```python
from build123d import *

# Parameters (mm, degrees)
SKETCH1_R           = 4.7625
BOSS_EXTRUDE1_DEPTH = 3.175
FILLET1_R           = 9.525


with BuildPart() as part:
    # Sketch1 → Boss-Extrude1 (new body)
    with BuildSketch(Plane.XY):
        Polygon((-195.314090033, 382.203190117), (-13.335, 248.156621006), (-13.335, 382.231468598), (-131.291653964, 469.118839915), align=None)
        with Locations((-35.56, 302.837639338)):
            Circle(SKETCH1_R, mode=Mode.SUBTRACT)
        with Locations((-35.56, 347.287639338)):
            Circle(SKETCH1_R, mode=Mode.SUBTRACT)
        with BuildLine():
            ThreePointArc((-154.070332508, 400.720749088), (-154.902423133, 400.218314877), (-155.846074695, 400.451417162))
            Line((-155.846074695, 400.451417162), (-161.470028505, 404.594045378))
            ThreePointArc((-161.470028505, 404.594045378), (-161.972462717, 405.426136003), (-161.739360431, 406.369787565))
            Line((-161.739360431, 406.369787565), (-129.351539832, 450.338880992))
            ThreePointArc((-129.351539832, 450.338880992), (-128.519449207, 450.841315204), (-127.575797645, 450.608212918))
            Line((-127.575797645, 450.608212918), (-121.951843834, 446.465584702))
            ThreePointArc((-121.951843834, 446.465584702), (-121.449409623, 445.633494077), (-121.682511908, 444.689842516))
            Line((-121.682511908, 444.689842516), (-154.070332508, 400.720749088))
        make_face(mode=Mode.SUBTRACT)
        Polygon((-150.783558745, 373.062079232), (-109.357276582, 429.301617336), (-54.61, 388.974541337), (-54.61, 302.220228189), (-96.036282162, 332.735003232), align=None, mode=Mode.SUBTRACT)
    extrude(amount=BOSS_EXTRUDE1_DEPTH)

    # Fillet1
    fillet1_edges = [part.edges().sort_by_distance(p)[0] for p in [
        (-54.61, 388.974541337, 1.5875),
        (-109.357276582, 429.301617336, 1.5875),
        (-150.783558745, 373.062079232, 1.5875),
        (-54.61, 302.220228189, 1.5875),
        (-131.291653964, 469.118839915, 1.5875),
        (-13.335, 382.231468598, 1.5875),
        (-13.335, 248.156621006, 1.5875),
        (-195.314090033, 382.203190117, 1.5875),
    ]]
    fillet(fillet1_edges, radius=FILLET1_R)


solid = part.part
```
Build history of the part. All positions in model axes, mm. A direction names the side the tool comes from. Round coordinates to 2 decimals unless told otherwise and drop trailing zeros. Write each loop counter-clockwise with the first axis right and the second up, starting at its lowest first coordinate (ties: lowest second). Pieces come first, ordered by that corner, then holes. Notation, with made-up numbers: (89, -18.75) - (128, -18.75) arc R23 cw to (128, -7.75) - close; hole circle Ø1 at (-24.5, -22.75). An arc over 180 degrees is marked (long way). Write each question's results on one line, items separated by ' | '. Start each with the question number.
Item 1: Drop a flat-ended pin along its axis: P1, Ø1.5, axis at x = -77.5, z = 1.5, coming from the +Y side. Give the stop position or say it passes through.
Item 2: Saw through at C-C (z = 2.5). State how many separate pieces and enclosed holes the cut face has, and give its area (3 significant figures).
Item 3: Saw through at B-B (x = -35.56). Write the cut outline in (y, z) (1 decimal), and give its area (3 significant figures).
Item 4: Which spindle directions (+Z, -Z, +X, -X, +Y, -Y) get a long thin tool onto all of the face, cutting with end or side? Do faces 1 (the face through (-158.619, 402.494, 1.565)), 2 (the face through (-18.695, 258.437, 1.61)). Say none if no direction does.
Item 5: Saw through at A-A (y = 364.5). Write the cut outline in (x, z) (3 decimals), and give its area (3 significant figures).
Item 6: Wall check: L1, parallel to X at y = 413, z = 1.4; L2, parallel to Y at x = -35.56, z = 0.9; L3, parallel to Y at x = -35, z = 2. Give the ranges that are in metal, low to high. Write a range as [from, to].
Results are:
1) P1: stops at y = 430.05
2) separate pieces: 1 | enclosed holes: 4 | area: 12,900 mm²
3) outline: (264.5, 0) - (298.1, 0) - (298.1, 3.2) - (264.5, 3.2) - close; (307.6, 0) - (342.5, 0) - (342.5, 3.2) - (307.6, 3.2) - close; (352.1, 0) - (398.6, 0) - (398.6, 3.2) - (352.1, 3.2) - close | area: 365 mm²
4) face 1: +Z, -Z | face 2: +Z, -Z, -Y
5) outline: (-171.281, 0) - (-139.16, 0) - (-139.16, 3.175) - (-171.281, 3.175) - close; (-54.61, 0) - (-13.335, 0) - (-13.335, 3.175) - (-54.61, 3.175) - close | area: 233 mm²
6) L1: x = [-172.63, -156.86], [-145.03, -121.37], [-87.23, -55.11] | L2: y = [264.53, 298.08], [307.6, 342.53], [352.05, 398.6] | L3: y = [264.12, 298.11], [307.57, 342.56], [352.02, 398.19]
